Here's how the part is built. I have some questions about the finished solid (model axes, mm). A direction names the side the tool comes from. Coordinates: 2 decimals unless noted, no trailing zeros. Loops run counter-clockwise (first coordinate to the right, second up) from the corner with the lowest first, then second, coordinate; pieces in that order, holes last. Notation, with made-up numbers: (9, 39) -> (14, 39) arc R19 cw to (14, 57) -> close; hole circle Ø1 at (86.25, 33). An arc over 180 degrees is marked (long way). Answer as a JSON object with one key per item and string values. Group by question number.
1) I want a section at B-B (x = 0). Write out the boundary of the cut face in (y, z).
2) Which directions (+Z, -Z, +X, -X, +Y, -Y) give clear straight access to the entire face, cutting with the end or side of a thin tool? Please do faces 4 (the flat face through (0, 46.5, 0)), 5 (the flat face through (0, 0, 0)), 6 (the cylindrical face through (-29.7, 81.3, 15.5)).
3) I want a section at D-D (x = 20.5). Write out the boundary of the cut face in (y, z), then the cut area to 3 significant figures.
4) I want a section at A-A (z = 0). Write out the boundary of the cut face in (x, y).
5) I want a section at C-C (y = 7). Write out the boundary of the cut face in (x, z).
6) I need wall thicknesses on probe 1 along X at (y, z) = (36.5, 0); probe 2 along X at (y, z) = (68, 0); probe 3 along Y at (x, z) = (-22.5, -17). Which ranges of each line are inside material? Lowest first, please. Write a range as [from, to].
7) I'm going to push flat-ended pins straight in: pin 1 (12 mm diameter, centred on x = 9.5, y = 67.5, fed in from -Z); pin 2 (2 mm diameter, centred on x = 12, z = 8, fed in from +Y); pin 3 (8 mm diameter, centred on y = 31, z = -1.5, fed in from +X). Where does each tip first touch, or does it pass through?
8) If we mould it in two halves opening along X, with no side actions, what happens to faces 1 (the cylindrical face through (7.81, 22.99, 1.73)), 2 (the cylindrical face through (3.955, 24.19, 5.158)), 3 (the flat face through (-34, 115, 0))? For each: +X half, -X half, draft (parallel to the pull), parting line (faces both ways), or undercut.
```python
from build123d import *

# Parameters (mm, degrees)
SKETCH1_R           = 8
BOSS_EXTRUDE1_DEPTH = 45
CHAMFER1_SIZE       = 3
CHAMFER1_SIZE2      = 1.595128295
SKETCH2_R           = 35
BOSS_EXTRUDE2_DEPTH = 70
SHELL1_T            = -1.5
SKETCH3_R           = 33.5
BOSS_EXTRUDE3_DEPTH = 2


with BuildPart() as part:
    # Sketch1 → Boss-Extrude1 (new body)
    with BuildSketch(Plane(origin=(0, 0, 0), x_dir=(1, 0, 0), z_dir=(0, 1, 0))):
        with Locations(Location((0, 0, 0), (0, 0, 90))):
            Circle(SKETCH1_R)
    extrude(amount=BOSS_EXTRUDE1_DEPTH)

    # Chamfer1
    chamfer1_edges = [part.edges().sort_by_distance(p)[0] for p in [
        (0, 0, 8),
    ]]
    chamfer1_side = [part.faces().sort_by_distance(p)[0] for p in [
        (0, 0, 0),
    ]]
    chamfer(chamfer1_edges, length=CHAMFER1_SIZE, length2=CHAMFER1_SIZE2, reference=chamfer1_side[0])

    # Sketch2 → Boss-Extrude2 (add)
    with BuildSketch(Plane(origin=(0, 45, 0), x_dir=(1, 0, 0), z_dir=(0, 1, 0))):
        with Locations(Location((0, 0, 0), (0, 0, 270))):
            Circle(SKETCH2_R)
    extrude(amount=BOSS_EXTRUDE2_DEPTH)

    # Shell1
    shell1_openings = [part.faces().sort_by_distance(p)[0] for p in [
        (0, 115, 0),
    ]]
    offset(amount=SHELL1_T, openings=shell1_openings, kind=Kind.INTERSECTION)

    # Sketch3 → Boss-Extrude3 (add)
    with BuildSketch(Plane(origin=(0, 46.5, 0), x_dir=(1, 0, 0), z_dir=(0, 1, 0))):
        with Locations(Location((0, 0, 0), (0, 0, 270))):
            Circle(SKETCH3_R)
    extrude(amount=BOSS_EXTRUDE3_DEPTH)


solid = part.part
```
Determined:
{
 "1": {"outline": "(0, -5) -> (1.6, -8) -> (45, -8) -> (45, -35) -> (115, -35) -> (115, -33.5) -> (48.5, -33.5) -> (48.5, 33.5) -> (115, 33.5) -> (115, 35) -> (45, 35) -> (45, 8) -> (1.6, 8) -> (0, 5) -> close; hole (1.5, -4.63) -> (2.5, -6.5) -> (46.5, -6.5) -> (46.5, 6.5) -> (2.5, 6.5) -> (1.5, 4.63) -> close"},
 "2": {"face 4": "none", "face 5": "+Z, -Z, +X, -X, -Y", "face 6": "+Y"},
 "3": {"outline": "(45, -28.37) -> (115, -28.37) -> (115, -26.5) -> (48.5, -26.5) -> (48.5, 26.5) -> (115, 26.5) -> (115, 28.37) -> (45, 28.37) -> close", "area": "448 mm^2"},
 "4": {"outline": "(-35, 45) -> (-8, 45) -> (-8, 1.6) -> (-5, 0) -> (5, 0) -> (8, 1.6) -> (8, 45) -> (35, 45) -> (35, 115) -> (33.5, 115) -> (33.5, 48.5) -> (-33.5, 48.5) -> (-33.5, 115) -> (-35, 115) -> close; hole (-6.5, 2.5) -> (-4.63, 1.5) -> (4.63, 1.5) -> (6.5, 2.5) -> (6.5, 46.5) -> (-6.5, 46.5) -> close"},
 "5": {"outline": "circle Ø16 at (0, 0); hole circle Ø13 at (0, 0)"},
 "6": {"probe 1": "[-8, -6.5], [6.5, 8]", "probe 2": "[-35, -33.5], [33.5, 35]", "probe 3": "[45, 48.5]"},
 "7": {"pin 1": "z = -34.82", "pin 2": "y = 48.5", "pin 3": "x = 8"},
 "8": {"face 1": "parting line", "face 2": "undercut", "face 3": "draft"}
}
